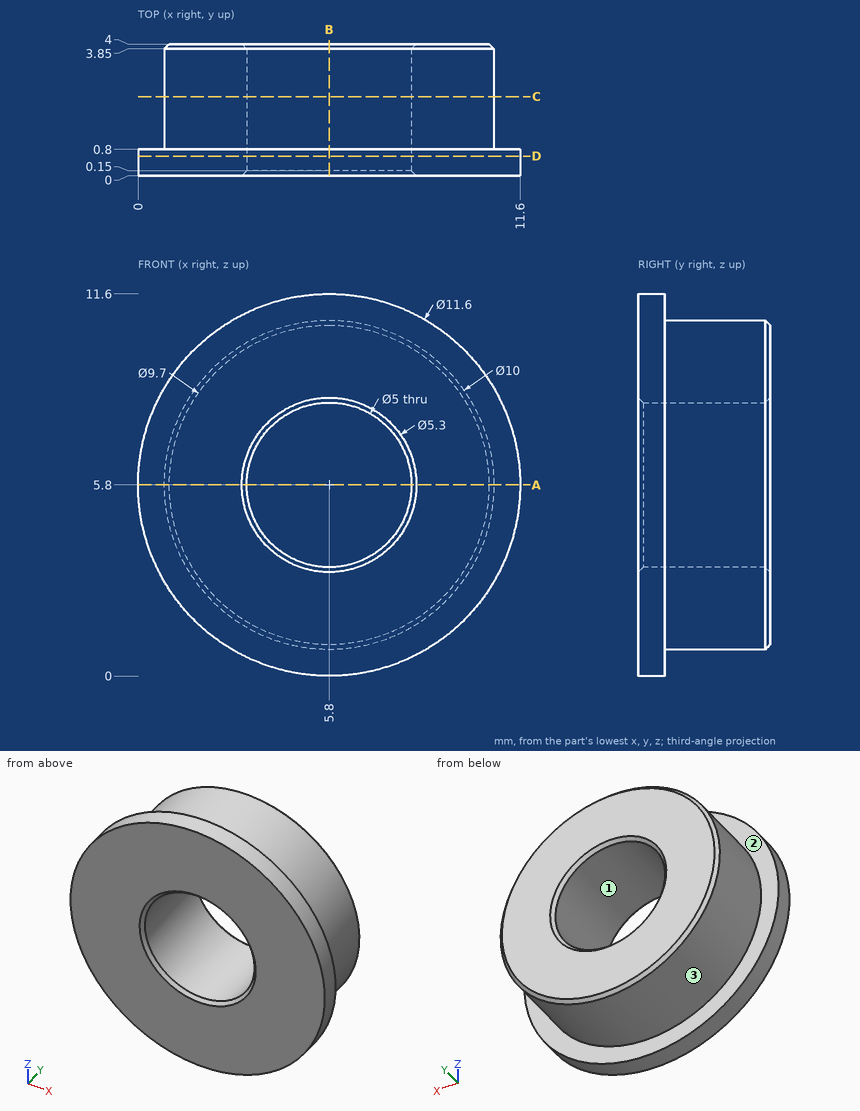
Print and shaded views of the part. All mm, measured from the part's lowest x, y and z. Round coordinates to 2 decimals unless told otherwise and drop trailing zeros. Write each loop counter-clockwise with the first axis right and the second up, starting at its lowest first coordinate (ties: lowest second). Pieces come first, ordered by that corner, then holes. Notation, with made-up numbers: (65, 19.5) -> (110, 19.5) arc R27 ccw to (110, 36.5) -> close; hole circle Ø11 at (75.5, 38.5). An arc over 180 degrees is marked (long way). Return JSON: item names as keys, results as strings. Group by question number.
Q1. Probe L1, parallel to X at y = 1.6, z = 5.8; L2, parallel to Y at x = 1.25, z = 3.5. List the from-to ranges inside material, lowest first. Write a range as [from, to].
Q2. Pin check, flat tips, straight feed: pin 1 (2 mm diameter, centred on y = 2.5, z = 4, fed in from -X); pin 2 (2 mm diameter, centred on x = 2.5, y = 2.5, fed in from -Z); pin 3 (1 mm diameter, centred on y = 2.5, z = 10.5, fed in from -X). Stop position of each tip, or through.
Q3. Saw through at D-D on y = 0.6. Write the cut outline in (x, z), plus the area to 3 significant figures.
Q4. Saw through at B-B on x = 5.8. Write the cut outline in (y, z), plus the area to 3 significant figures.
Q5. Mould opens along Z. For the marked faces 1, 2 and 3 say: pulls with the +Z half, pulls with the -Z half, needs draft (parallel to the pull), parting line crosses it, or undercut.
Q6. Saw through at C-C on y = 2.4. Write the cut outline in (x, z), plus the area to 3 significant figures.
Q7. Saw through at A-A on z = 5.8. Write the cut outline in (x, y).
Answer:
{
 "1": {"L1": "[0.8, 3.3], [8.3, 10.8]", "L2": "[0, 0.8]"},
 "2": {"pin 1": "x = 0.86", "pin 2": "z = 1.36", "pin 3": "x = 3.09"},
 "3": {"outline": "circle Ø11.6 at (5.8, 5.8); hole circle Ø5 at (5.8, 5.8)", "area": "86.0 mm2"},
 "4": {"outline": "(0, 0) -> (0.8, 0) -> (0.8, 0.8) -> (3.85, 0.8) -> (4, 0.95) -> (4, 3.15) -> (3.85, 3.3) -> (0.15, 3.3) -> (0, 3.15) -> close; (0, 8.45) -> (0.15, 8.3) -> (3.85, 8.3) -> (4, 8.45) -> (4, 10.65) -> (3.85, 10.8) -> (0.8, 10.8) -> (0.8, 11.6) -> (0, 11.6) -> close", "area": "21.2 mm2"},
 "5": {"face 1": "undercut", "face 2": "needs draft", "face 3": "parting line crosses it"},
 "6": {"outline": "circle Ø10 at (5.8, 5.8); hole circle Ø5 at (5.8, 5.8)", "area": "58.9 mm2"},
 "7": {"outline": "(0, 0) -> (3.15, 0) -> (3.3, 0.15) -> (3.3, 3.85) -> (3.15, 4) -> (0.95, 4) -> (0.8, 3.85) -> (0.8, 0.8) -> (0, 0.8) -> close; (8.3, 0.15) -> (8.45, 0) -> (11.6, 0) -> (11.6, 0.8) -> (10.8, 0.8) -> (10.8, 3.85) -> (10.65, 4) -> (8.45, 4) -> (8.3, 3.85) -> close"}
}
